Geometry: final body of the model. Coordinates: model frame, mm. Face numbers are marked on the shaded views. A direction names the side the tool comes from. Give positions to 0.01 mm unless a question says otherwise; leave off trailing zeros. Write each loop counter-clockwise with the first axis right and the second up, starting at its lowest first coordinate (ties: lowest second). Pieces come first, ordered by that corner, then holes.
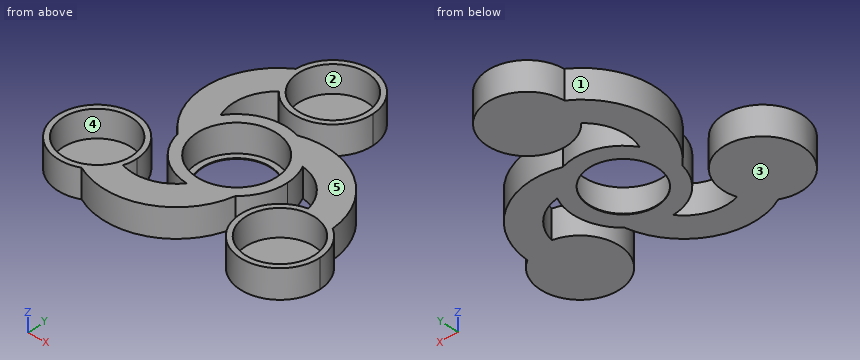
```python
from build123d import *

# Parameters (mm, degrees)
F1_DEPTH = 8
F2_R     = 9.6
F3_DEPTH = 7.5
F4_R     = 9.5
F5_DEPTH = 8
F6_R     = 11.075
F7_DEPTH = 7.8


with BuildPart() as f1:
    # F0 (on Top) → F1 (new body)
    with BuildSketch(Plane.XY):
        with BuildLine():
            ThreePointArc((-20.338538175, -24.4089821655), (-2.1146153157, -24.8073076343), (9.2222039848, -10.5333258595))
            ThreePointArc((9.2222039848, -10.5333258595), (4.4593163175, -13.2708137648), (-0.9901909161, -13.9649390242))
            ThreePointArc((-0.9901909161, -13.9649390242), (-7.2029967728, -18.2136446038), (-14.7291218144, -18.1247763029))
            ThreePointArc((-14.7291218144, -18.1247763029), (-16.9084612176, -21.8250967603), (-20.338538175, -24.4089821655))
        make_face()
        with BuildLine():
            ThreePointArc((9.2222039848, -10.5333258595), (12.7497226595, -5.7831282284), (14, 0))
            ThreePointArc((14, 0), (13.6427127767, 3.1426721262), (12.5890874153, 6.1249390242))
            ThreePointArc((12.5890874153, 6.1249390242), (5.35662199, 4.9902566208), (0, 0))
            ThreePointArc((0, 0), (1.64337801, -7.1340990322), (-0.9901909161, -13.9649390242))
            ThreePointArc((-0.9901909161, -13.9649390242), (4.4593163175, -13.2708137648), (9.2222039848, -10.5333258595))
        make_face()
        with BuildLine():
            ThreePointArc((-0.9901909161, -13.9649390242), (1.64337801, -7.1340990322), (0, 0))
            ThreePointArc((0, 0), (-7, 2.1438424114), (-11.5988964992, 7.84))
            ThreePointArc((-11.5988964992, 7.84), (-13.722520008, 2.773525668), (-13.7332297731, -2.72))
            ThreePointArc((-13.7332297731, -2.72), (-9.2632036905, -10.4972880968), (-0.9901909161, -13.9649390242))
        make_face()
        with BuildLine():
            ThreePointArc((-14.1147367097, -14.5), (-34.4297295676, -8.6492814066), (-20.338538175, -24.4089821655))
            ThreePointArc((-20.338538175, -24.4089821655), (-16.9084612176, -21.8250967603), (-14.7291218144, -18.1247763029))
            ThreePointArc((-14.7291218144, -18.1247763029), (-14.2694205814, -16.3382377637), (-14.1147367097, -14.5))
        make_face()
        with BuildLine():
            ThreePointArc((31.3080677234, -5.4091996526), (27.3553188432, -3.7306085732), (23.0610776234, -3.6934055153))
            ThreePointArc((23.0610776234, -3.6934055153), (18.100118044, -22.9732003974), (36.1147367097, -14.5))
            ThreePointArc((36.1147367097, -14.5), (34.8391040709, -9.3583388458), (31.3080677234, -5.4091996526))
        make_face()
        with BuildLine():
            ThreePointArc((4.5110257882, 13.2533258595), (9.2632036905, 10.4972880968), (12.5890874153, 6.1249390242))
            ThreePointArc((12.5890874153, 6.1249390242), (19.3749773088, 2.8688441133), (23.0610776234, -3.6934055153))
            ThreePointArc((23.0610776234, -3.6934055153), (27.3553188432, -3.7306085732), (31.3080677234, -5.4091996526))
            ThreePointArc((31.3080677234, -5.4091996526), (22.5410662686, 10.5723432345), (4.5110257882, 13.2533258595))
        make_face()
        with BuildLine():
            ThreePointArc((0, 0), (5.35662199, 4.9902566208), (12.5890874153, 6.1249390242))
            ThreePointArc((12.5890874153, 6.1249390242), (9.2632036905, 10.4972880968), (4.5110257882, 13.2533258595))
            ThreePointArc((4.5110257882, 13.2533258595), (-4.4593163175, 13.2708137648), (-11.5988964992, 7.84))
            ThreePointArc((-11.5988964992, 7.84), (-7, 2.1438424114), (0, 0))
        make_face()
        with BuildLine():
            ThreePointArc((-13.7332297731, -2.72), (-13.722520008, 2.773525668), (-11.5988964992, 7.84))
            ThreePointArc((-11.5988964992, 7.84), (-12.171980536, 15.3448004906), (-8.331955809, 21.8181818182))
            ThreePointArc((-8.331955809, 21.8181818182), (-10.4468576256, 25.5557053335), (-10.9695295484, 29.8181818182))
            ThreePointArc((-10.9695295484, 29.8181818182), (-20.4264509529, 14.2349643998), (-13.7332297731, -2.72))
        make_face()
        with BuildLine():
            ThreePointArc((-10.9695295484, 29.8181818182), (-10.4468576256, 25.5557053335), (-8.331955809, 21.8181818182))
            ThreePointArc((-8.331955809, 21.8181818182), (3.8306974627, 18.6885618389), (11, 29))
            ThreePointArc((11, 29), (0.4093745034, 39.9923797476), (-10.9695295484, 29.8181818182))
        make_face()
    extrude(amount=F1_DEPTH)

    # F2 (on face) → F3 (cut)
    with BuildSketch(Plane.XY.offset(8)):
        with Locations((0, 29)):
            Circle(F2_R)
        with Locations((-25.1147367097, -14.5)):
            Circle(F2_R)
        with Locations((25.1147367097, -14.5)):
            Circle(F2_R)
    extrude(amount=-F3_DEPTH, mode=Mode.SUBTRACT)

    # F4 (on face) → F5 (cut, through all)
    with BuildSketch(Plane.XY.offset(8)):
        Circle(F4_R)
    extrude(amount=-F5_DEPTH, mode=Mode.SUBTRACT)

    # F6 (on face) → F7 (cut)
    with BuildSketch(Plane.XY.offset(8)):
        Circle(F6_R)
    extrude(amount=-F7_DEPTH, mode=Mode.SUBTRACT)


solid = f1.part
```
Item 1: Pull-direction query (X, two-part tool) for the marked faces 1, 2 and 3; classes: +X half, -X half, draft (parallel to the pull), parting line (faces both ways), or undercut.
Found:
face 1: -X half
face 2: undercut
face 3: draft
Item 2: Pin query (flat end, axial travel): pin 1 Ø22 at (x, y) = (25.11, -14.5) entering from -Z; pin 2 Ø8 at (x, y) = (16.5, 18) entering from -Z; pin 3 Ø6 at (x, y) = (0.5, 25.5) entering from +Z; pin 4 Ø4 at (y, z) = (-3, 5) entering from -X. Return the tip coordinate at first contact, or that it passes through.
Found:
pin 1: stops at z = 0
pin 2: passes through
pin 3: stops at z = 0.5
pin 4: stops at x = -30.66
Item 3: Reachability of the marked faces 4 and 5 from +Z, -Z, +X, -X, +Y, -Y: full face, straight path, thin tool, end or side. Return the list, or none.
Found:
face 4: +Z
face 5: +Z, +X, -X, +Y, -Y
Item 4: Section A-A, the plane x = -19. Return the cut outline in (y, z).
Found:
outline: (-25.05, 0) - (-5.36, 0) - (-5.36, 8) - (-7.1, 8) - (-7.1, 0.5) - (-21.9, 0.5) - (-21.9, 8) - (-25.05, 8) - close; (4.8, 0) - (20.2, 0) - (20.2, 8) - (4.8, 8) - close
Item 5: Section D-D, the plane y = 31. Return the cut outline in (x, z).
Found:
outline: (-10.82, 0) - (10.82, 0) - (10.82, 8) - (9.39, 8) - (9.39, 0.5) - (-9.39, 0.5) - (-9.39, 8) - (-10.82, 8) - close
Item 6: Section C-C, the plane z = 6.25. Return the cut outline in (x, y) (3 decimals), plus the area to 3 significant figures.
Found:
outline: (-20.339, -24.409) arc R20.5 ccw to (9.222, -10.533) arc R14 ccw to (12.589, 6.125) arc R12.5 cw to (23.061, -3.693) arc R11 ccw (long way) to (31.308, -5.409) arc R20.5 ccw to (4.511, 13.253) arc R14 ccw to (-11.599, 7.84) arc R12.5 cw to (-8.332, 21.818) arc R11 ccw (long way) to (-10.97, 29.818) arc R20.5 ccw to (-13.733, -2.72) arc R14 ccw to (-0.99, -13.965) arc R12.5 cw to (-14.729, -18.125) arc R11 ccw (long way) to start; hole circle Ø19.2 at (-25.115, -14.5); hole circle Ø22.15 at (0, 0); hole circle Ø19.2 at (0, 29); hole circle Ø19.2 at (25.115, -14.5)
area: 1,110 mm2
Item 7: Line query: L1, parallel to X at y = -17, z = 4.75; L2, parallel to X at y = -7, z = 7.25; L3, parallel to X at y = 3, z = 2. Output: solid intervals per line, ascending.
Found:
L1: x = -35.83 to -34.38, -15.85 to -14.4, -4.45 to 6.63, 14.4 to 15.85, 34.38 to 35.83
L2: x = -33.16 to -31.11, -19.12 to -17.07, -12.12 to -8.58, 8.58 to 12.12, 17.07 to 19.12, 31.11 to 33.16
L3: x = -18.17 to -10.66, 10.66 to 13.67, 19.23 to 29.12
Item 8: Section B-B, the plane x = 0. Return the cut outline in (y, z) (3 decimals).
Found:
outline: (-23.659, 0) - (-9.5, 0) - (-9.5, 0.2) - (-11.075, 0.2) - (-11.075, 8) - (-23.659, 8) - close; (9.5, 0) - (14, 0) - (14, 8) - (11.075, 8) - (11.075, 0.2) - (9.5, 0.2) - close; (18, 0) - (40, 0) - (40, 8) - (38.6, 8) - (38.6, 0.5) - (19.4, 0.5) - (19.4, 8) - (18, 8) - close
